Verification items for the finished model (mm, model axes). Coordinates: 2 decimals unless noted, no trailing zeros. Order: outer loops, then holes, each group sorted by start corner. A loop starts at its lowest first (then second) coordinate and runs counter-clockwise, first axis right, second up. Notation, with made-up numbers: (86.25, -1) -> (113.25, -1) arc R8 ccw to (113.25, 13) -> close; hole circle Ø7 at (57, -38). An arc over 180 degrees is marked (long way). Answer as CSV lines item,"result".
```python
from build123d import *

# Parameters (mm, degrees)
SKETCH1_R           = 12.5
SKETCH1_R_2         = 2.55
BOSS_EXTRUDE1_DEPTH = 3


with BuildPart() as part:
    # Sketch1 → Boss-Extrude1 (new body)
    with BuildSketch(Plane(origin=(0, 0, 0), x_dir=(1, 0, 0), z_dir=(0, 1, 0))):
        with BuildLine():
            Line((15.75, -60.75), (-15.75, -60.75))
            ThreePointArc((-15.75, -60.75), (-18.578427125, -59.578427125), (-19.75, -56.75))
            Line((-19.75, -56.75), (-19.75, 17.25))
            ThreePointArc((-19.75, 17.25), (-18.578427125, 20.078427125), (-15.75, 21.25))
            Line((-15.75, 21.25), (15.75, 21.25))
            ThreePointArc((15.75, 21.25), (18.578427125, 20.078427125), (19.75, 17.25))
            Line((19.75, 17.25), (19.75, -56.75))
            ThreePointArc((19.75, -56.75), (18.578427125, -59.578427125), (15.75, -60.75))
        make_face()
        Circle(SKETCH1_R, mode=Mode.SUBTRACT)
        with Locations((10, -52.55)):
            Circle(SKETCH1_R_2, mode=Mode.SUBTRACT)
        with Locations((10, -32.55)):
            Circle(SKETCH1_R_2, mode=Mode.SUBTRACT)
        with Locations((0, -52.55)):
            Circle(SKETCH1_R_2, mode=Mode.SUBTRACT)
        with Locations((0, -32.55)):
            Circle(SKETCH1_R_2, mode=Mode.SUBTRACT)
        with Locations((-10, -52.55)):
            Circle(SKETCH1_R_2, mode=Mode.SUBTRACT)
        with Locations((-10, -32.55)):
            Circle(SKETCH1_R_2, mode=Mode.SUBTRACT)
        with BuildLine():
            Line((11.903984489, 14.096015511), (14.403984489, 16.596015511))
            ThreePointArc((14.403984489, 16.596015511), (16.596015511, 16.596015511), (16.596015511, 14.403984489))
            Line((16.596015511, 14.403984489), (14.096015511, 11.903984489))
            ThreePointArc((14.096015511, 11.903984489), (11.903984489, 11.903984489), (11.903984489, 14.096015511))
        make_face(mode=Mode.SUBTRACT)
        with BuildLine():
            Line((-11.903984489, 14.096015511), (-14.403984489, 16.596015511))
            ThreePointArc((-14.403984489, 16.596015511), (-16.596015511, 16.596015511), (-16.596015511, 14.403984489))
            Line((-16.596015511, 14.403984489), (-14.096015511, 11.903984489))
            ThreePointArc((-14.096015511, 11.903984489), (-11.903984489, 11.903984489), (-11.903984489, 14.096015511))
        make_face(mode=Mode.SUBTRACT)
        with BuildLine():
            Line((-11.903984489, -14.096015511), (-14.403984489, -16.596015511))
            ThreePointArc((-14.403984489, -16.596015511), (-16.596015511, -16.596015511), (-16.596015511, -14.403984489))
            Line((-16.596015511, -14.403984489), (-14.096015511, -11.903984489))
            ThreePointArc((-14.096015511, -11.903984489), (-11.903984489, -11.903984489), (-11.903984489, -14.096015511))
        make_face(mode=Mode.SUBTRACT)
        with BuildLine():
            Line((11.903984489, -14.096015511), (14.403984489, -16.596015511))
            ThreePointArc((14.403984489, -16.596015511), (16.596015511, -16.596015511), (16.596015511, -14.403984489))
            Line((16.596015511, -14.403984489), (14.096015511, -11.903984489))
            ThreePointArc((14.096015511, -11.903984489), (11.903984489, -11.903984489), (11.903984489, -14.096015511))
        make_face(mode=Mode.SUBTRACT)
    extrude(amount=BOSS_EXTRUDE1_DEPTH)


solid = part.part
```
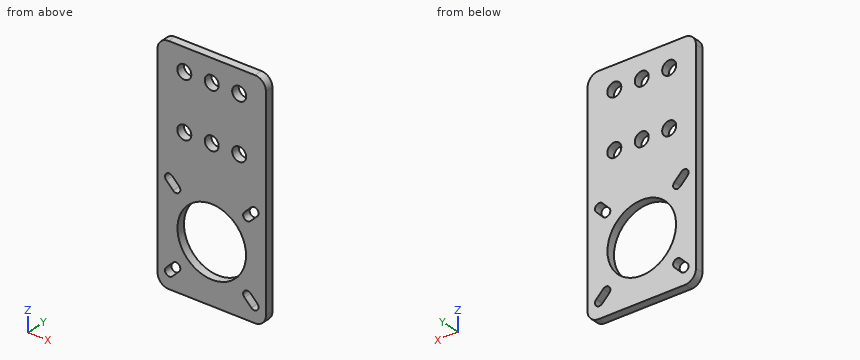
Item 1: Section check C-C, the plane z = 32.55. Record the boundary of the cut face in (x, y), plus the area to 3 significant figures.
Answer list:
outline,"(-19.75, 0) -> (-12.55, 0) -> (-12.55, 3) -> (-19.75, 3) -> close; (-7.45, 0) -> (-2.55, 0) -> (-2.55, 3) -> (-7.45, 3) -> close; (2.55, 0) -> (7.45, 0) -> (7.45, 3) -> (2.55, 3) -> close; (12.55, 0) -> (19.75, 0) -> (19.75, 3) -> (12.55, 3) -> close"
area,"72.6 mm2"
Item 2: Section check A-A, the plane x = 3.5. Record the boundary of the cut face in (y, z).
Answer list:
outline,"(0, -21.25) -> (3, -21.25) -> (3, -12) -> (0, -12) -> close; (0, 12) -> (3, 12) -> (3, 60.75) -> (0, 60.75) -> close"
Item 3: Section check D-D, the plane z = 0. Record the boundary of the cut face in (x, y).
Answer list:
outline,"(-19.75, 0) -> (-12.5, 0) -> (-12.5, 3) -> (-19.75, 3) -> close; (12.5, 0) -> (19.75, 0) -> (19.75, 3) -> (12.5, 3) -> close"
Item 4: Section check B-B, the plane y = 0.5. Count the separate pieces of the cut face and the enclosed holes in it, plus the area to 3 significant figures.
Answer list:
separate pieces,"1"
enclosed holes,"11"
area,"2,540 mm2"
Item 5: Depth check by flat-ended pin: pin 1 Ø6.5 at (x, z) = (10, 32.55) entering from -Y. Enter the tip coordinate at first touch or a pass-through.
Answer list:
pin 1,"y = 0"
Item 6: Thickness scan on line 1 (X direction, y = 1.3, z = 32.55); line 2 (Z direction, x = 0, y = 2.2); line 3 (Z direction, x = -16, y = 0.7). Record the ranges inside material, lowest first.
Answer list:
line 1,"-19.75 to -12.55, -7.45 to -2.55, 2.55 to 7.45, 12.55 to 19.75"
line 2,"-21.25 to -12.5, 12.5 to 30, 35.1 to 50, 55.1 to 60.75"
line 3,"-21.24 to -16.97, -13.81 to 13.81, 16.97 to 60.74"
